from build123d import *

# Parameters (mm, degrees)
SKETCH1_R           = 1.143
SKETCH1_W           = 5.08
SKETCH1_H           = 3.175
BOSS_EXTRUDE1_DEPTH = 2.54
FILLET1_R           = 1.27


with BuildPart() as part:
    # Sketch1 → Boss-Extrude1 (new body)
    with BuildSketch(Plane(origin=(0, 0, 0), x_dir=(1, 0, 0), z_dir=(0, 1, 0))):
        with BuildLine():
            Line((-27.94, 13.208), (-27.94, -13.208))
            Line((-27.94, -13.208), (-27.178, -13.208))
            Line((-27.178, -13.208), (-7.509126714, -13.208))
            ThreePointArc((-7.509126714, -13.208), (0, -8.382), (7.509126714, -13.208))
            Line((7.509126714, -13.208), (27.178, -13.208))
            Line((27.178, -13.208), (27.94, -13.208))
            Line((27.94, -13.208), (27.94, 13.208))
            Line((27.94, 13.208), (-27.94, 13.208))
        make_face()
        with BuildLine():
            Line((-7.509126714, -13.208), (-27.178, -13.208))
            Line((-27.178, -13.208), (-27.178, -18.542))
            Line((-27.178, -18.542), (-15.0495, -18.542))
            Line((-15.0495, -18.542), (-9.9695, -18.542))
            Line((-9.9695, -18.542), (-9.9695, -14.224))
            Line((-9.9695, -14.224), (-7.894457296, -14.224))
            ThreePointArc((-7.894457296, -14.224), (-7.718527326, -13.709652922), (-7.509126714, -13.208))
        make_face()
        with Locations((-11.8745, -16.637)):
            Circle(SKETCH1_R, mode=Mode.SUBTRACT)
        with BuildLine():
            Line((27.178, -13.208), (7.509126714, -13.208))
            ThreePointArc((7.509126714, -13.208), (7.718527326, -13.709652922), (7.894457296, -14.224))
            Line((7.894457296, -14.224), (9.9695, -14.224))
            Line((9.9695, -14.224), (9.9695, -18.542))
            Line((9.9695, -18.542), (15.0495, -18.542))
            Line((15.0495, -18.542), (27.178, -18.542))
            Line((27.178, -18.542), (27.178, -13.208))
        make_face()
        with Locations((11.8745, -16.637)):
            Circle(SKETCH1_R, mode=Mode.SUBTRACT)
        with Locations((-12.5095, -20.1295)):
            Rectangle(SKETCH1_W, SKETCH1_H)
        with Locations((12.5095, -20.1295)):
            Rectangle(SKETCH1_W, SKETCH1_H)
    extrude(amount=BOSS_EXTRUDE1_DEPTH)

    # Fillet1
    fillet1_edges = [part.edges().sort_by_distance(p)[0] for p in [
        (15.0495, 1.27, 18.542),
        (-15.0495, 1.27, 18.542),
    ]]
    fillet(fillet1_edges, radius=FILLET1_R)


solid = part.part
Verification items for the finished model (mm, model axes). A direction names the side the tool comes from. Round coordinates to 2 decimals unless told otherwise and drop trailing zeros. Order: outer loops, then holes, each group sorted by start corner. A loop starts at its lowest first (then second) coordinate and runs counter-clockwise, first axis right, second up. Notation, with made-up numbers: (10, 75) -> (69, 75) arc R23 cw to (69, 112) -> close; hole circle Ø7 at (69, 15.5). An arc over 180 degrees is marked (long way). Put each result on its own line as item: value.
1) Section check C-C (x = 23.5). Record the cut outline in (y, z).
Final values:
outline: (0, -13.21) -> (2.54, -13.21) -> (2.54, 18.54) -> (0, 18.54) -> close
2) Mould release check, pull along X, two halves, no side actions. Record for faces 4 (the flat face through (-9, 1, 14.224)), 5 (the flat face through (-9.97, 1, 18)), 6 (the cylindrical face through (-15.431, 1.288, 18.904)), 7 (the flat face through (0, 2.54, 0)): +X half, -X half, draft (parallel to the pull), parting line (faces both ways), or undercut.
Final values:
face 4: undercut
face 5: undercut
face 6: -X half
face 7: draft
3) Section check B-B (y = 0.45). Record the cut outline in (x, z) (1 decimal).
Final values:
outline: (-27.9, -13.2) -> (27.9, -13.2) -> (27.9, 13.2) -> (27.2, 13.2) -> (27.2, 18.5) -> (16.3, 18.5) arc R1.3 cw to (15, 19.8) -> (15, 21.7) -> (10, 21.7) -> (10, 14.2) -> (7.9, 14.2) arc R8.3 cw to (-7.9, 14.2) -> (-10, 14.2) -> (-10, 21.7) -> (-15, 21.7) -> (-15, 19.8) arc R1.3 cw to (-16.3, 18.5) -> (-27.2, 18.5) -> (-27.2, 13.2) -> (-27.9, 13.2) -> close; hole circle Ø2.3 at (-11.9, 16.6); hole circle Ø2.3 at (11.9, 16.6)
4) Section check A-A (z = 12). Record the cut outline in (x, y).
Final values:
outline: (-27.94, 0) -> (-6.83, 0) -> (-6.83, 2.54) -> (-27.94, 2.54) -> close; (6.83, 0) -> (27.94, 0) -> (27.94, 2.54) -> (6.83, 2.54) -> close
5) Section check D-D (x = -9). Record the cut outline in (y, z), then the cut area to 3 significant figures.
Final values:
outline: (0, -13.21) -> (2.54, -13.21) -> (2.54, 14.22) -> (0, 14.22) -> close
area: 69.7 mm^2
6) Depth check by flat-ended pin: pin 1 (1.3 mm diameter, centred on x = -20.5, y = 1, fed in from +Z); pin 2 (4 mm diameter, centred on x = -13, z = -9.5, fed in from -Y); pin 3 (2 mm diameter, centred on x = 11.87, z = 16.64, fed in from +Y); pin 4 (0.6 mm diameter, centred on y = 1, z = 20.5, fed in from -X). Enter the tip coordinate at first touch or a pass-through.
Final values:
pin 1: stops at z = 18.54
pin 2: stops at y = 0
pin 3: passes through
pin 4: stops at x = -15.05
7) Set-up check for faces 1 (the flat face through (15.049, 1, 21)), 2 (the flat face through (9, 1, 14.224)), 3 (the flat face through (-15.049, 1, 21)): record each of +Z, -Z, +X, -X, +Y, -Y from which the full face is reachable in a straight line by a thin tool's end or side.
Final values:
face 1: +Z, +X, +Y, -Y
face 2: +Z, +Y, -Y
face 3: +Z, -X, +Y, -Y
8) Material ranges on line 1 (Z direction, x = 12, y = 0.75); line 2 (X direction, y = 0.85, z = 14.5); line 3 (X direction, y = 0.1, z = 20), recorded low to high.
Final values:
line 1: z = -13.21 to 15.5, 17.77 to 21.72
line 2: x = -27.18 to -9.97, 9.97 to 27.18
line 3: x = -15.05 to -9.97, 9.97 to 15.05
